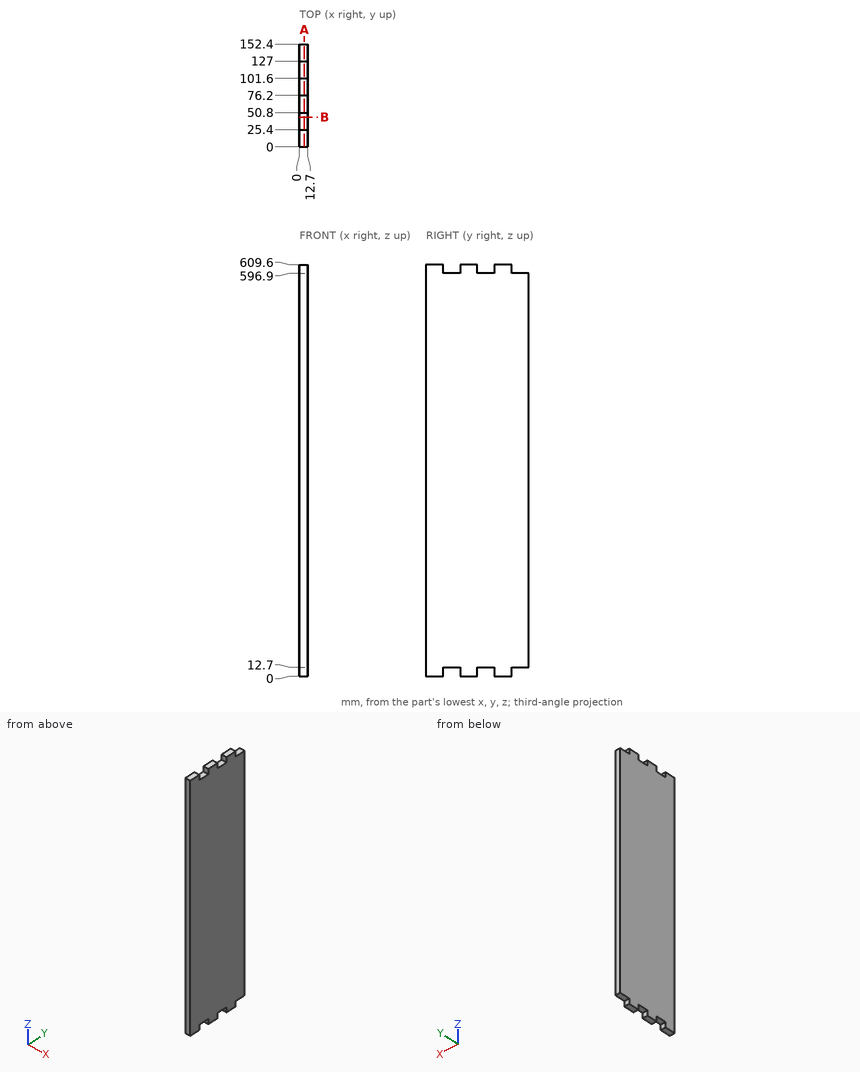
Design review of the part shown in the three views and the two pictorial views. Dimensions are in mm from the part's minimum x, y and z. Coordinates: 2 decimals unless noted, no trailing zeros. Order: outer loops, then holes, each group sorted by start corner. A loop starts at its lowest first (then second) coordinate and runs counter-clockwise, first axis right, second up. Notation, with made-up numbers: (-6.75, -5.75) -> (3.25, -5.75) arc R27 cw to (3.25, 16.25) -> close; hole circle Ø6 at (68.25, -38.75). An arc over 180 degrees is marked (long way). Use one line per item in the form item = value. Start each with the question number.
(1) Insertion check: pin 1 (6.5 mm diameter, centred on x = 7.5, z = 5, fed in from +Y); pin 2 (4 mm diameter, centred on x = 4, y = 136, fed in from +Z); pin 3 (6.5 mm diameter, centred on x = 8, z = 5.5, fed in from -Y); pin 4 (4 mm diameter, centred on x = 5.5, y = 90.5, fed in from -Z). Each pin has a flat end and moves straight along its axis. Give the tip position at first contact, or say it passes through.
(2) Add section B-B on y = 44. State the section outline as (x, z) points, plus the area to 3 significant figures.
(3) Add section A-A on x = 7.5. State the section outline as (y, z) points.
(4) For probe 1 along Z at (x, y) = (10, 40), list the stretches that pass through material, from the lowest coordinate up.
Answer block:
q1.pin_1 = 127
q1.pin_2 = 596.9
q1.pin_3 = 0
q1.pin_4 = 12.7
q2.outline = (0, 12.7) -> (12.7, 12.7) -> (12.7, 596.9) -> (0, 596.9) -> close
q2.area = 7,420 mm²
q3.outline = (0, 0) -> (25.4, 0) -> (25.4, 12.7) -> (50.8, 12.7) -> (50.8, 0) -> (76.2, 0) -> (76.2, 12.7) -> (101.6, 12.7) -> (101.6, 0) -> (127, 0) -> (127, 12.7) -> (152.4, 12.7) -> (152.4, 596.9) -> (127, 596.9) -> (127, 609.6) -> (101.6, 609.6) -> (101.6, 596.9) -> (76.2, 596.9) -> (76.2, 609.6) -> (50.8, 609.6) -> (50.8, 596.9) -> (25.4, 596.9) -> (25.4, 609.6) -> (0, 609.6) -> close
q4.probe_1 = 12.7 to 596.9
